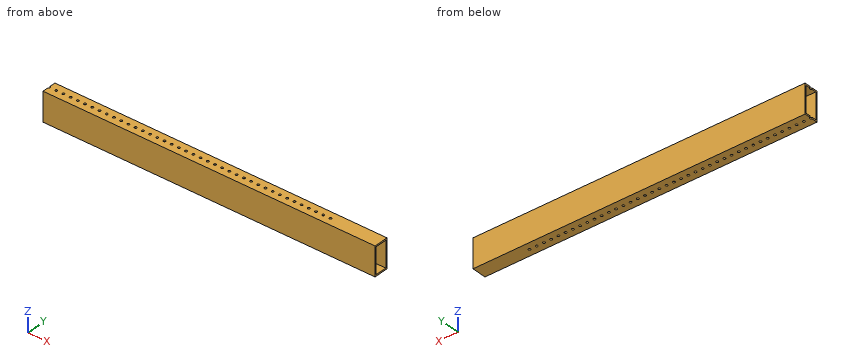
from build123d import *

# Parameters (mm, degrees)
SKETCH1_W           = 50.8
SKETCH1_H           = 25.4
SKETCH1_W_2         = 45.72
SKETCH1_H_2         = 20.32
BOSS_EXTRUDE1_DEPTH = 292.1
SKETCH2_R           = 2.032
CUT_EXTRUDE1_DEPTH  = 297.756364717


with BuildPart() as part:
    # Sketch1 → Boss-Extrude1 (new, symmetric)
    with BuildSketch(Plane(origin=(0, 0, 0), x_dir=(0, 0, -1), z_dir=(1, 0, 0))):
        Rectangle(SKETCH1_W, SKETCH1_H)
        Rectangle(SKETCH1_W_2, SKETCH1_H_2, mode=Mode.SUBTRACT)
    extrude(amount=BOSS_EXTRUDE1_DEPTH, both=True)

    # Sketch2 → Cut-Extrude1 (cut, through all)
    with BuildSketch(Plane.XY.offset(25.4)):
        with Locations((-292.1, 0)):
            Circle(SKETCH2_R)
        with Locations((-279.4, 0)):
            Circle(SKETCH2_R)
        with Locations((-266.7, 0)):
            Circle(SKETCH2_R)
        with Locations((-254, 0)):
            Circle(SKETCH2_R)
        with Locations((-241.3, 0)):
            Circle(SKETCH2_R)
        with Locations((-228.6, 0)):
            Circle(SKETCH2_R)
        with Locations((-215.9, 0)):
            Circle(SKETCH2_R)
        with Locations((-203.2, 0)):
            Circle(SKETCH2_R)
        with Locations((-190.5, 0)):
            Circle(SKETCH2_R)
        with Locations((-177.8, 0)):
            Circle(SKETCH2_R)
        with Locations((-165.1, 0)):
            Circle(SKETCH2_R)
        with Locations((-152.4, 0)):
            Circle(SKETCH2_R)
        with Locations((-139.7, 0)):
            Circle(SKETCH2_R)
        with Locations((-127, 0)):
            Circle(SKETCH2_R)
        with Locations((-114.3, 0)):
            Circle(SKETCH2_R)
        with Locations((-101.6, 0)):
            Circle(SKETCH2_R)
        with Locations((-88.9, 0)):
            Circle(SKETCH2_R)
        with Locations((-76.2, 0)):
            Circle(SKETCH2_R)
        with Locations((-63.5, 0)):
            Circle(SKETCH2_R)
        with Locations((-50.8, 0)):
            Circle(SKETCH2_R)
        with Locations((-38.1, 0)):
            Circle(SKETCH2_R)
        with Locations((-25.4, 0)):
            Circle(SKETCH2_R)
        with Locations((-12.7, 0)):
            Circle(SKETCH2_R)
        Circle(SKETCH2_R)
        with Locations((12.7, 0)):
            Circle(SKETCH2_R)
        with Locations((25.4, 0)):
            Circle(SKETCH2_R)
        with Locations((38.1, 0)):
            Circle(SKETCH2_R)
        with Locations((50.8, 0)):
            Circle(SKETCH2_R)
        with Locations((63.5, 0)):
            Circle(SKETCH2_R)
        with Locations((76.2, 0)):
            Circle(SKETCH2_R)
        with Locations((88.9, 0)):
            Circle(SKETCH2_R)
        with Locations((101.6, 0)):
            Circle(SKETCH2_R)
        with Locations((114.3, 0)):
            Circle(SKETCH2_R)
        with Locations((127, 0)):
            Circle(SKETCH2_R)
        with Locations((139.7, 0)):
            Circle(SKETCH2_R)
        with Locations((152.4, 0)):
            Circle(SKETCH2_R)
        with Locations((165.1, 0)):
            Circle(SKETCH2_R)
        with Locations((177.8, 0)):
            Circle(SKETCH2_R)
        with Locations((190.5, 0)):
            Circle(SKETCH2_R)
        with Locations((203.2, 0)):
            Circle(SKETCH2_R)
    extrude(amount=-CUT_EXTRUDE1_DEPTH, mode=Mode.SUBTRACT)


solid = part.part
The model under review builds one solid part; all positions refer to its coordinate system, in mm. Round coordinates to 2 decimals unless told otherwise and drop trailing zeros. Write each loop counter-clockwise with the first axis right and the second up, starting at its lowest first coordinate (ties: lowest second). Pieces come first, ordered by that corner, then holes. Notation, with made-up numbers: (8, -19) -> (15, -19) arc R23 ccw to (15, 3) -> close; hole circle Ø6 at (53, -29.75). An arc over 180 degrees is marked (long way). Answer as a JSON object with one key per item and string values.
1. To check wall thickness, follow line 1 along Z through (x, y) = (-100, 2.75); line 2 along Y through (x, z) = (113.5, 5); line 3 along Y through (x, z) = (190, -23). State the ranges of each line that lie inside material, in increasing order.
Results found:
{"line 1": "z = -25.4 to -22.86, 22.86 to 25.4", "line 2": "y = -12.7 to -10.16, 10.16 to 12.7", "line 3": "y = -12.7 to -1.97, 1.97 to 12.7"}
2. Clearance check with a flat-ended pin moving along its axis: pin 1 (2.5 mm diameter, centred on x = 114.3, y = 0, fed in from -Z). State where the tip first meets the part, or that it passes through.
Results found:
{"pin 1": "passes through"}
3. We need section A-A on z = -3. State the section outline as (x, y) points, and give its area (3 significant figures).
Results found:
{"outline": "(-292.1, -12.7) -> (292.1, -12.7) -> (292.1, -10.16) -> (-292.1, -10.16) -> close; (-292.1, 10.16) -> (292.1, 10.16) -> (292.1, 12.7) -> (-292.1, 12.7) -> close", "area": "2,970 mm^2"}
